```python
from build123d import *

# Parameters (mm, degrees)
CYLINDER001_R     = 2.5
CYLINDER001_DEPTH = 10


with BuildPart() as cone001:
    # Cone001 → Cone001 (revolve)
    with BuildSketch(Plane(origin=(0, 0, -3), x_dir=(1, 0, 0), z_dir=(0, -1, 0))):
        Polygon((0, 0), (4.5, 0), (2.5, 3), (0, 3), align=None)
    revolve(axis=Axis((0, 0, -3), (0, 0, 1)))


with BuildPart() as obj1:
    # Cylinder001 → Cylinder001 (new body)
    with BuildSketch(Plane.XY):
        Circle(CYLINDER001_R)
    extrude(amount=CYLINDER001_DEPTH)

    # Fusion001: union Cone001
    add(cone001.part)


solid = obj1.part
```
Geometry: final body of the model. Coordinates: model frame, mm. A direction names the side the tool comes from. Coordinates: 2 decimals unless noted, no trailing zeros. Order: outer loops, then holes, each group sorted by start corner. A loop starts at its lowest first (then second) coordinate and runs counter-clockwise, first axis right, second up. Notation, with made-up numbers: (16, 23) - (62, 23) arc R31 ccw to (62, 55) - close; hole circle Ø10 at (-20.5, 47.25). An arc over 180 degrees is marked (long way). Write each question's results on one line, items separated by ' | '.
1) Section A-A, the plane y = 0. Return loops of the section in (x, z).
Results list:
outline: (-4.5, -3) - (4.5, -3) - (2.5, 0) - (2.5, 10) - (-2.5, 10) - (-2.5, 0) - close
2) Set-up query: faces 1 (the cylindrical face through (-0.54, -2.44, 4.93)), 2 (the flat face through (0, 0, 10)). Return all of +Z, -Z, +X, -X, +Y, -Y with unobstructed straight access to the full face (end or side cutting, diameter ignored); none if empty.
Results list:
face 1: +Z | face 2: +Z, +X, -X, +Y, -Y
3) Section C-C, the plane z = -1.25. Return loops of the section in (x, y), plus the area to 3 significant figures.
Results list:
outline: circle Ø6.67 at (0, 0) | area: 34.9 mm^2
4) Pin query (flat end, axial travel): pin 1 (2 mm diameter, centred on x = 1, z = 8.5, fed in from +Y); pin 2 (5 mm diameter, centred on x = 2, z = 5.5, fed in from -Y); pin 3 (5 mm diameter, centred on y = 3.5, z = -0.5, fed in from +X). Return the tip coordinate at first contact, or that it passes through.
Results list:
pin 1: y = 2.5 | pin 2: y = -2.5 | pin 3: x = 3.66
5) Section D-D, the plane z = 4. Return loops of the section in (x, y).
Results list:
outline: circle Ø5 at (0, 0)
6) Line query: line 1 (Z direction, x = -0.5, y = 4.25); line 2 (X direction, y = -0.5, z = 5). Output: solid intervals per line, ascending. Write a range as from..to.
Results list:
line 1: -3..-2.67 | line 2: -2.45..2.45
